```python
from build123d import *

# Parameters (mm, degrees)
SKETCH1_W           = 304.8
SKETCH1_H           = 25.4
BOSS_EXTRUDE2_DEPTH = 12.7
FILLET1_R           = 12.7
CUT_EXTRUDE3_DEPTH  = 281.209703849
SKETCH8_W           = 70
SKETCH8_H           = 25.4
BOSS_EXTRUDE3_DEPTH = 9.7
CUT_EXTRUDE4_DEPTH  = 281.209703849
CUT_EXTRUDE5_DEPTH  = 281.209703849
SKETCH13_W          = 12.7
SKETCH13_H          = 25.4
CUT_EXTRUDE7_DEPTH  = 280.450243045


with BuildPart() as part:
    # Sketch1 → Boss-Extrude2 (new body)
    with BuildSketch(Plane.XY):
        with Locations((126.366978193, -2.136448598)):
            Rectangle(SKETCH1_W, SKETCH1_H)
    extrude(amount=BOSS_EXTRUDE2_DEPTH)

    # Fillet1
    fillet1_edges = [part.edges().sort_by_distance(p)[0] for p in [
        (-26.033021807, -2.136448598, 12.7),
        (278.766978193, -2.136448598, 12.7),
    ]]
    fillet(fillet1_edges, radius=FILLET1_R - 0.0001)  # a hair under: the kernel refuses the full size

    # Sketch6 → Cut-Extrude3 (cut, through all)
    with BuildSketch(Plane(origin=(0, 10.563551402, 0), x_dir=(1, 0, 0), z_dir=(0, 1, 0))):
        with BuildLine():
            Line((-23.033021807, 0), (275.766978193, 0))
            ThreePointArc((275.766978193, 0), (272.925913971, -6.858935778), (266.066978193, -9.7))
            Line((266.066978193, -9.7), (-13.333021807, -9.7))
            ThreePointArc((-13.333021807, -9.7), (-20.191957584, -6.858935778), (-23.033021807, 0))
        make_face()
    extrude(amount=-CUT_EXTRUDE3_DEPTH, mode=Mode.SUBTRACT)

    # Sketch8 → Boss-Extrude3 (add)
    with BuildSketch(Plane(origin=(0, 0, 9.7), x_dir=(-1, 0, 0), z_dir=(0, 0, -1))):
        with Locations((-180.266978193, -2.136448598)):
            Rectangle(SKETCH8_W, SKETCH8_H)
        with Locations((-72.466978193, -2.136448598)):
            Rectangle(SKETCH8_W, SKETCH8_H)
    extrude(amount=BOSS_EXTRUDE3_DEPTH)

    # Sketch9 → Cut-Extrude4 (cut, through all)
    with BuildSketch(Plane(origin=(0, 10.563551402, 0), x_dir=(1, 0, 0), z_dir=(0, 1, 0))):
        Polygon((145.266978193, -9.7), (165.266978193, -9.7), (192.266978193, -9.7), (165.266978193, -3), (145.266978193, -3), align=None)
        Polygon((215.266978193, -6.7), (195.266978193, -6.7), (168.266978193, 0), (215.266978193, 0), align=None)
    extrude(amount=-CUT_EXTRUDE4_DEPTH, mode=Mode.SUBTRACT)

    # Sketch12 → Cut-Extrude5 (cut, through all)
    with BuildSketch(Plane(origin=(0, 10.563551402, 0), x_dir=(1, 0, 0), z_dir=(0, 1, 0))):
        Polygon((107.466978193, -9.7), (107.466978193, -3), (87.466978193, -3), (60.466978193, -9.7), align=None)
        Polygon((37.466978193, -6.7), (57.466978193, -6.7), (84.466978193, 0), (37.466978193, 0), align=None)
    extrude(amount=-CUT_EXTRUDE5_DEPTH, mode=Mode.SUBTRACT)

    # Sketch13 → Cut-Extrude7 (cut, through all)
    with BuildSketch(Plane.XY.offset(12.7)):
        with Locations((-19.683021807, -2.136448598)):
            Rectangle(SKETCH13_W, SKETCH13_H)
        with Locations((272.416978193, -2.136448598)):
            Rectangle(SKETCH13_W, SKETCH13_H)
    extrude(amount=-CUT_EXTRUDE7_DEPTH, mode=Mode.SUBTRACT)


solid = part.part
```
Geometry: final body of the model. Coordinates: model frame, mm. A direction names the side the tool comes from. Round coordinates to 2 decimals unless told otherwise and drop trailing zeros. Loops run counter-clockwise (first coordinate to the right, second up) from the corner with the lowest first, then second, coordinate; pieces in that order, holes last.
Item 1: Section A-A, the plane x = 97. Output: boundary loops of the cut face in (y, z).
Checked values:
outline: (-14.84, 0) - (10.56, 0) - (10.56, 3) - (-14.84, 3) - close; (-14.84, 9.7) - (10.56, 9.7) - (10.56, 12.7) - (-14.84, 12.7) - close
Item 2: Section D-D, the plane x = 64.5. Output: boundary loops of the cut face in (y, z), plus the area to 3 significant figures.
Checked values:
outline: (-14.84, 4.95) - (10.56, 4.95) - (10.56, 8.7) - (-14.84, 8.7) - close; (-14.84, 9.7) - (10.56, 9.7) - (10.56, 12.7) - (-14.84, 12.7) - close
area: 171 mm2
Item 3: Mould query, pull axis X, two halves, no side actions, for faces 1 (the flat face through (178.956, -1.959, 6.397)), 2 (the flat face through (125, -2, 9.7)), 3 (the flat face through (126, -14.836, 11)), 4 (the flat face through (181.956, -1.959, 3.397)). Classes: released by +X, released by -X, zero draft, split by the parting line, or undercut.
Checked values:
face 1: undercut
face 2: undercut
face 3: zero draft
face 4: released by +X
Item 4: Section C-C, the plane x = 230. Output: boundary loops of the cut face in (y, z).
Checked values:
outline: (-14.84, 9.7) - (10.56, 9.7) - (10.56, 12.7) - (-14.84, 12.7) - close
Item 5: Contact query for flat-ended pins moving along their axis: P1, Ø12, axis at x = 210, y = -3, coming from the -Z side; P2, Ø7.5, axis at x = 233, y = 1, coming from the -Z side; P3, Ø4, axis at x = 34, z = 5.5, coming from the -Y side (1 decimal); P4, Ø5, axis at y = -3.5, z = 9, coming from the +X side. Output: stop coordinate, or through.
Checked values:
P1: stops at z = 6.7
P2: stops at z = 9.7
P3: passes through
P4: stops at x = 266.07
Item 6: Line query: L1, parallel to Z at x = 103.5, y = -10.5; L2, parallel to Z at x = 189.5, y = 7.25; L3, parallel to Z at x = 19.5, y = -4.75. Output: solid intervals per line, ascending.
Checked values:
L1: z = 0 to 3, 9.7 to 12.7
L2: z = 5.27 to 9.01, 9.7 to 12.7
L3: z = 9.7 to 12.7
Item 7: Reachability of faces 5 (the flat face through (12, -2, 9.7)), 6 (the flat face through (155, -2, 3)), 7 (the flat face through (205, -2, 6.7)), 8 (the flat face through (126, 10.564, 11)) from +Z, -Z, +X, -X, +Y, -Y: full face, straight path, thin tool, end or side. Return the list, or none.
Checked values:
face 5: -Z, -X, +Y, -Y
face 6: +Y, -Y
face 7: -Z, +X, +Y, -Y
face 8: +Z, -Z, +X, -X, +Y
Item 8: Section B-B, the plane y = -11.5. Output: boundary loops of the cut face in (x, z).
Checked values:
outline: (-13.33, 9.7) - (37.47, 9.7) - (37.47, 6.7) - (57.47, 6.7) - (84.47, 0) - (107.47, 0) - (107.47, 3) - (87.47, 3) - (60.47, 9.7) - (192.27, 9.7) - (165.27, 3) - (145.27, 3) - (145.27, 0) - (168.27, 0) - (195.27, 6.7) - (215.27, 6.7) - (215.27, 9.7) - (266.07, 9.7) - (266.07, 12.7) - (-13.33, 12.7) - close
